```python
from build123d import *

# Parameters (mm, degrees)
SKETCH1_R           = 25.4
BOSS_EXTRUDE1_DEPTH = 44.45
SKETCH2_R           = 79.375
BOSS_EXTRUDE2_DEPTH = 2.4003
SKETCH3_R           = 79.375
SKETCH3_R_2         = 71.755
BOSS_EXTRUDE3_DEPTH = 0.5461
SKETCH4_R           = 39.624
BOSS_EXTRUDE4_DEPTH = 0.5461
SKETCH5_R           = 4.7625
CUT_EXTRUDE1_DEPTH  = 122.849086919


with BuildPart() as part:
    # Sketch1 → Boss-Extrude1 (new body)
    with BuildSketch(Plane(origin=(0, 0, 0), x_dir=(0, 0, -1), z_dir=(1, 0, 0))):
        Circle(SKETCH1_R)
    boss_extrude1 = extrude(amount=BOSS_EXTRUDE1_DEPTH)

    # Sketch2 → Boss-Extrude2 (add)
    with BuildSketch(Plane(origin=(44.45, 0, 0), x_dir=(0, 0, -1), z_dir=(1, 0, 0))):
        Circle(SKETCH2_R)
    boss_extrude2 = extrude(amount=BOSS_EXTRUDE2_DEPTH)

    # Sketch3 → Boss-Extrude3 (add)
    with BuildSketch(Plane(origin=(46.8503, 0, 0), x_dir=(0, 0, -1), z_dir=(1, 0, 0))):
        Circle(SKETCH3_R)
        Circle(SKETCH3_R_2, mode=Mode.SUBTRACT)
    boss_extrude3 = extrude(amount=BOSS_EXTRUDE3_DEPTH)

    # Sketch4 → Boss-Extrude4 (add)
    with BuildSketch(Plane(origin=(46.8503, 0, 0), x_dir=(0, 0, -1), z_dir=(1, 0, 0))):
        Circle(SKETCH4_R)
    boss_extrude4 = extrude(amount=BOSS_EXTRUDE4_DEPTH)

    # Sketch5 → Cut-Extrude1 (cut, through all)
    with BuildSketch(Plane(origin=(47.3964, 0, 0), x_dir=(0, 0, -1), z_dir=(1, 0, 0))):
        Circle(SKETCH5_R)
    cut_extrude1 = extrude(amount=-CUT_EXTRUDE1_DEPTH, mode=Mode.SUBTRACT)

    # Mirror1: Boss-Extrude1, Boss-Extrude2, Boss-Extrude3, Boss-Extrude4, Cut-Extrude1 across plane
    add(boss_extrude1.mirror(Plane(origin=(0, 0, 0), x_dir=(0, 0, 1), z_dir=(1, 0, 0))))
    add(boss_extrude2.mirror(Plane(origin=(0, 0, 0), x_dir=(0, 0, 1), z_dir=(1, 0, 0))))
    add(boss_extrude3.mirror(Plane(origin=(0, 0, 0), x_dir=(0, 0, 1), z_dir=(1, 0, 0))))
    add(boss_extrude4.mirror(Plane(origin=(0, 0, 0), x_dir=(0, 0, 1), z_dir=(1, 0, 0))))
    add(cut_extrude1.mirror(Plane(origin=(0, 0, 0), x_dir=(0, 0, 1), z_dir=(1, 0, 0))), mode=Mode.SUBTRACT)


solid = part.part
```
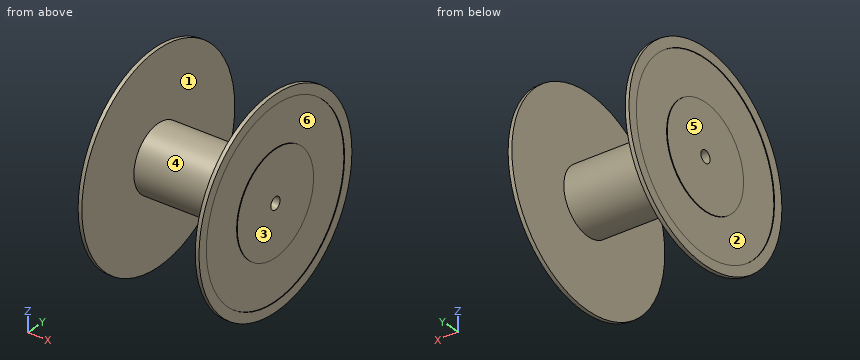
The model under review builds one solid part; all positions refer to its coordinate system, in mm. Face numbers are marked on the shaded views. A direction names the side the tool comes from. Coordinates: 2 decimals unless noted, no trailing zeros. Write each loop counter-clockwise with the first axis right and the second up, starting at its lowest first coordinate (ties: lowest second). Pieces come first, ordered by that corner, then holes.
1) Clearance check with flat-ended pins moving along their axes: pin 1 Ø6 at (x, y) = (-6, -1.5) entering from -Z; pin 2 Ø8 at (x, z) = (32, 7.5) entering from +Y; pin 3 Ø5 at (x, y) = (-20, -22.5) entering from +Z. State where each tip first meets the part, or that it passes through.
2) We need section D-D on y = 37.5. State the section outline as (x, z) points, then the cut area to 3 significant figures.
3) We need section C-C on x = 27. State the section outline as (y, z) points (1 decimal), then the cut area to 3 significant figures.
4) Machinability: for the marked faces 1, 2 and 3, which of the approach directions +Z, -Z, +X, -X, +Y, -Y give a long, thin tool a straight path to every point of the face, cutting with its end or side? Answer none if there is none.
5) The part is to be moulded in two halves that separate along Z. For the marked faces 4, 5 and 6, say which applies: pulls with the +Z half, pulls with the -Z half, needs draft (parallel to the pull), parting line crosses it, or undercut.
6) To check wall thickness, follow probe 1 along Y at (x, z) = (-47, 0) (1 decimal); probe 2 along X at (y, z) = (19.5, 57); probe 3 along X at (y, z) = (4.5, 32.5). State the ranges of each line that lie inside material, in increasing order.
Answer list:
1. pin 1: stops at z = -25.4
1. pin 2: stops at y = 25.16
1. pin 3: stops at z = 15.66
2. outline: (-47.4, -69.96) - (-44.45, -69.96) - (-44.45, 69.96) - (-47.4, 69.96) - (-47.4, 61.18) - (-46.85, 61.18) - (-46.85, 12.8) - (-47.4, 12.8) - (-47.4, -12.8) - (-46.85, -12.8) - (-46.85, -61.18) - (-47.4, -61.18) - close; (44.45, -69.96) - (47.4, -69.96) - (47.4, -61.18) - (46.85, -61.18) - (46.85, -12.8) - (47.4, -12.8) - (47.4, 12.8) - (46.85, 12.8) - (46.85, 61.18) - (47.4, 61.18) - (47.4, 69.96) - (44.45, 69.96) - close
2. area: 719 mm2
3. outline: circle Ø50.8 at (0, 0); hole circle Ø9.5 at (0, 0)
3. area: 1,960 mm2
4. face 1: none
4. face 2: -X
4. face 3: +Z, -Z, +X, +Y, -Y
5. face 4: parting line crosses it
5. face 5: needs draft
5. face 6: undercut
6. probe 1: y = -79.4 to -71.8, -39.6 to -4.8, 4.8 to 39.6, 71.8 to 79.4
6. probe 2: x = -46.85 to -44.45, 44.45 to 46.85
6. probe 3: x = -47.4 to -44.45, 44.45 to 47.4
